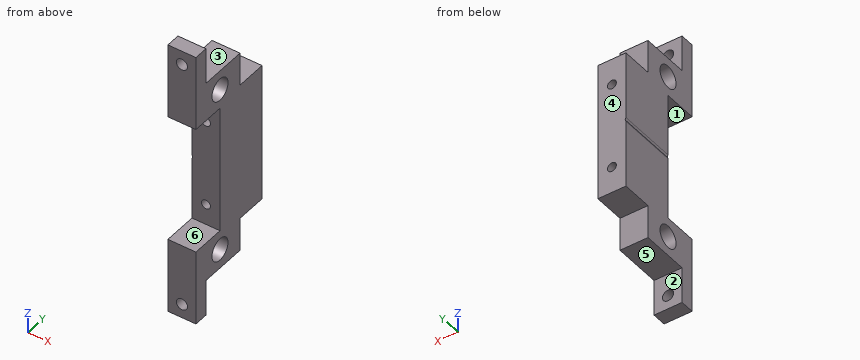
Autodesk Inventor part; units mm, degrees
ref_plane "YZ Plane" through (0, 0, 0) normal (1, 0, 0) x (0, 1, 0)
ref_plane "XZ Plane" through (0, 0, 0) normal (0, 1, 0) x (-1, 0, 0)
ref_plane "XY Plane" through (0, 0, 0) normal (0, 0, 1) x (1, 0, 0)
sketch "Sketch1" plane through (0, 0, 0) normal (1, 0, 0) x (0, 1, 0)
  line L0 (0, 50) -> (0, 23)
  line L1 (0, 23) -> (12, 23)
  line L2 (12, 23) -> (12, -23)
  line L3 (12, -23) -> (0, -23)
  line L4 (0, -23) -> (0, -50)
  line L5 (0, -50) -> (5, -50)
  line L6 (5, -50) -> (5, -37)
  line L7 (5, -37) -> (22, -37)
  line L8 (22, -37) -> (22, -25)
  line L9 (22, -25) -> (33, -25)
  line L10 (33, -25) -> (33, 25)
  line L11 (33, 25) -> (22, 25)
  line L12 (22, 25) -> (22, 37)
  line L13 (22, 37) -> (5, 37)
  line L14 (5, 37) -> (5, 50)
  line L15 (5, 50) -> (0, 50)
  circle A0 centre (12, 30) radius 4
  circle A1 centre (12, -30) radius 4
  point P0 (0, 0)
  point P1 (12, 0)
  dimension "d0" = 100
  dimension "d1" = 46
  dimension "d2" = 27
  dimension "d3" = 5
  dimension "d4" = 17
  dimension "d5" = 13
  dimension "d6" = 12
  dimension "d7" = 11
  dimension "d8" = 12
  dimension "d9" = 8
  dimension "d10" = 30
  dimension "d11" = 30
  dimension "d12" = 12
extrude "Extrusion1" add sketch "Sketch1" along normal blind 10
sketch "Sketch2" plane through (0, 0, 23) normal (0, -1, 0) x (1, 0, 0)
  circle A0 centre (5, 22) radius 2
  circle A1 centre (5, -7.5) radius 1.6
  circle A2 centre (5, -38.5) radius 1.6
  circle A3 centre (5, -68) radius 2
  line L0 (0, 27) -> (10, 27)
  point P0 (0, -23)
  point P1 (5, 27)
  dimension "d15" = 4
  dimension "d16" = 3.2
  dimension "d17" = 15.5
  dimension "d18" = 15.5
  dimension "d19" = 90
  dimension "d20" = 45
extrude "Extrusion2" cut sketch "Sketch2" against normal through all
sketch "Sketch3" plane through (0, 33, 25) normal (0, 1, 0) x (1, 0, 0)
  line L0 (0.3, 25) -> (0, 25.72)
  line L1 (0, 50) -> (0, 0)
  line L2 (0, 24.28) -> (0.3, 25)
  point P0 (0, 25)
  point P1 (0, 25)
  dimension "d23" = 0.72
  dimension "d24" = 0.3
  dimension "d25" = 0.72
extrude "Extrusion3" cut sketch "Sketch3" against normal up to next
equation "\"d21\" = d18"
properties material "ABS Plastic"
Source: CAD feature listing. Evaluate the final solid. Frame: model axes, mm. Face numbers are marked on the shaded views. A direction names the side the tool comes from. Give positions to 0.01 mm unless a question says otherwise; leave off trailing zeros. Order: outer loops, then holes, each group sorted by start corner. A loop starts at its lowest first (then second) coordinate and runs counter-clockwise, first axis right, second up. Notation, with made-up numbers: (44, 16.25) -> (78, 16.25) arc R27 ccw to (78, 33.25) -> close; hole circle Ø9 at (-24, -16). An arc over 180 degrees is marked (long way). Use a Markdown table: item, result.
Q1. Material intervals for line 1 (Z direction, x = 5, y = 21.25); line 2 (Z direction, x = 5, y = 3.6); line 3 (Z direction, x = 5.25, y = 22.5), sorted ascending. Write a range as [from, to].
A:
| item | result |
|---|---|
| line 1 | [-37, -17.1], [-13.9, 13.9], [17.1, 37] |
| line 2 | [-50, -47], [-43, -23], [23, 43], [47, 50] |
| line 3 | [-25, -17.08], [-13.92, 13.92], [17.08, 25] |
Q2. Section B-B (x = 5). State how many separate pieces and enclosed holes the cut face has, and give its area (3 significant figures).
A:
| item | result |
|---|---|
| separate pieces | 5 |
| enclosed holes | 2 |
| area | 1,480 mm^2 |
Q3. Section C-C (y = 18). Return the cut outline in (x, z), and give its area (3 significant figures).
A:
| item | result |
|---|---|
| outline | (0, -37) -> (10, -37) -> (10, 37) -> (0, 37) -> (0, 0.72) -> (0.3, 0) -> (0, -0.72) -> close; hole circle Ø3.2 at (5, -15.5); hole circle Ø3.2 at (5, 15.5) |
| area | 724 mm^2 |
Q4. Section A-A (z = 45). Return the cut outline in (x, y).
A:
| item | result |
|---|---|
| outline | (0, 0) -> (3, 0) -> (3, 5) -> (0, 5) -> close; (7, 0) -> (10, 0) -> (10, 5) -> (7, 5) -> close |
Q5. Section D-D (y = 10). Return the cut outline in (x, z), and give its area (3 significant figures).
A:
| item | result |
|---|---|
| outline | (0, -37) -> (10, -37) -> (10, -33.46) -> (0, -33.46) -> close; (0, -26.54) -> (10, -26.54) -> (10, -23) -> (0, -23) -> close; (0, 23) -> (10, 23) -> (10, 26.54) -> (0, 26.54) -> close; (0, 33.46) -> (10, 33.46) -> (10, 37) -> (0, 37) -> close |
| area | 141 mm^2 |
Q6. Access query for the marked faces 1, 2 and 3. Directions: +Z, -Z, +X, -X, +Y, -Y. A direction counts if a zero-diameter tool reaches every point of the face in a straight line with its end or side. Return the directions, or none.
A:
| item | result |
|---|---|
| face 1 | +X, -X, -Y |
| face 2 | -Z, +X, -X, +Y |
| face 3 | +Z, +X, -X, +Y |
Q7. Pull-direction query (Z, two-part tool) for the marked faces 4, 5 and 6; classes: +Z half, -Z half, draft (parallel to the pull), parting line (faces both ways), or undercut.
A:
| item | result |
|---|---|
| face 4 | draft |
| face 5 | -Z half |
| face 6 | undercut |
Q8. First-contact query: P1, Ø5, axis at x = 1.5, y = 26.5, coming from the -Z side; P2, Ø5, axis at x = 2.5, z = -29, coming from the +Y side; P3, Ø3, axis at x = 5.5, y = 28, coming from the +Z side. Flat tips, straight axial feed; report the tip coordinate or a pass-through.
A:
| item | result |
|---|---|
| P1 | z = -25 |
| P2 | y = 22 |
| P3 | z = 25 |
